Could you check a few things on this model? Use its own coordinates, in mm. A direction names the side the tool comes from. Coordinates: 2 decimals unless noted, no trailing zeros. Write each loop counter-clockwise with the first axis right and the second up, starting at its lowest first coordinate (ties: lowest second). Pieces come first, ordered by that corner, then holes. Notation, with made-up numbers: (-16, 19) - (-11, 19) arc R22 ccw to (-11, 31) - close; hole circle Ø6 at (73, -1). An arc over 180 degrees is marked (long way). Write item = value, one per line. Start each with the question number.
```python
from build123d import *

# Parameters (mm, degrees)
SKETCH1_W           = 40
SKETCH1_H           = 40
BOSS_EXTRUDE1_DEPTH = 40
SKETCH2_W           = 10
SKETCH2_H           = 20
CUT_EXTRUDE1_DEPTH  = 40
CUT_EXTRUDE2_DEPTH  = 40
CUT_EXTRUDE3_DEPTH  = 40
CUT_EXTRUDE4_DEPTH  = 20
CUT_EXTRUDE5_DEPTH  = 10


with BuildPart() as part:
    # Sketch1 → Boss-Extrude1 (new body)
    with BuildSketch(Plane.XY):
        with Locations((20, 20)):
            Rectangle(SKETCH1_W, SKETCH1_H)
    extrude(amount=BOSS_EXTRUDE1_DEPTH)

    # Sketch2 → Cut-Extrude1 (cut)
    with BuildSketch(Plane.XY.offset(40)):
        with Locations((5, 30)):
            Rectangle(SKETCH2_W, SKETCH2_H)
    extrude(amount=-CUT_EXTRUDE1_DEPTH, mode=Mode.SUBTRACT)

    # Sketch3 → Cut-Extrude2 (cut)
    with BuildSketch(Plane.ZY.offset(-10)):
        with BuildLine():
            Line((0, 40), (0, 20))
            ThreePointArc((0, 20), (5.857864376, 34.142135624), (20, 40))
            Line((20, 40), (0, 40))
        make_face()
        with BuildLine():
            Line((40, 40), (20, 40))
            ThreePointArc((20, 40), (34.142135624, 34.142135624), (40, 20))
            Line((40, 20), (40, 40))
        make_face()
    extrude(amount=-CUT_EXTRUDE2_DEPTH, mode=Mode.SUBTRACT)

    # Sketch4 → Cut-Extrude3 (cut)
    with BuildSketch(Plane.ZY):
        with BuildLine():
            ThreePointArc((20, 0), (5.857864376, 5.857864376), (0, 20))
            Line((0, 20), (0, 0))
            Line((0, 0), (20, 0))
        make_face()
        with BuildLine():
            ThreePointArc((40, 20), (34.142135624, 5.857864376), (20, 0))
            Line((20, 0), (40, 0))
            Line((40, 0), (40, 20))
        make_face()
    extrude(amount=-CUT_EXTRUDE3_DEPTH, mode=Mode.SUBTRACT)

    # Sketch5 → Cut-Extrude4 (cut)
    with BuildSketch(Plane.ZY):
        with BuildLine():
            Line((20, 0), (20, 20))
            Line((20, 20), (40, 20))
            ThreePointArc((40, 20), (34.142135624, 5.857864376), (20, 0))
        make_face()
    extrude(amount=-CUT_EXTRUDE4_DEPTH, mode=Mode.SUBTRACT)

    # Sketch6 → Cut-Extrude5 (cut)
    with BuildSketch(Plane(origin=(40, 0, 0), x_dir=(0, 0, -1), z_dir=(1, 0, 0))):
        with BuildLine():
            Line((-20, 40), (-20, 0))
            ThreePointArc((-20, 0), (-40, 20), (-20, 40))
        make_face()
    extrude(amount=-CUT_EXTRUDE5_DEPTH, mode=Mode.SUBTRACT)


solid = part.part
```
1) Suppose I cut it at D-D on z = 4. Please give me the cut outline in (x, y), plus the area to 3 significant figures.
2) Suppose I cut it at A-A on z = 32. Please give me the cut outline in (x, y).
3) If I drill on probe 1 along X at (y, z) = (19, 38.5); probe 2 along Z at (x, y) = (13, 19.5); probe 3 along X at (y, z) = (31, 9.5), over which ranges is the centre line in solid material (lowest first)? Write a range as [from, to].
4) Suppose I cut it at B-B on x = 33.5. Please give me the cut outline in (y, z), plus the area to 3 significant figures.
5) Which directions (+Z, -Z, +X, -X, +Y, -Y) give clear straight access to the entire face, cutting with the end or side of a thin tool? Please do faces 1 (the flat face through (20, 12, 28)), 2 (the flat face through (10, 28, 20)), 3 (the flat face through (0, 12, 12)), 4 (the flat face through (30, 20, 28)), 5 (the flat face through (40, 20, 12)).
6) Suppose I cut it at C-C on y = 13. Please give me the cut outline in (x, z) (3 decimals).
7) For P1, Ø1.5, axis at y = 32.5, z = 23, coming from the +X side; P2, Ø5, axis at x = 14.5, z = 26, coming from the -Y side; P3, Ø6, axis at y = 11, z = 31, coming from the -X side, each with a flat end and sliding along its axis, tell me the tip position at first contact or that it passes through.
Reply:
q1.outline = (0, 8) - (40, 8) - (40, 32) - (10, 32) - (10, 20) - (0, 20) - close
q1.area = 840 mm^2
q2.outline = (10, 20) - (20, 20) - (20, 4) - (30, 4) - (30, 36) - (10, 36) - close
q3.probe_1 = [20, 30]
q3.probe_2 = [0.01, 20]
q3.probe_3 = [10, 40]
q4.outline = (0, 20) arc R20 ccw to (40, 20) - close
q4.area = 628 mm^2
q5.face_1 = +Z, -X, -Y
q5.face_2 = +Z, -Z, -X, +Y
q5.face_3 = +Z, -Z, -X, +Y, -Y
q5.face_4 = +Z, +X, +Y, -Y
q5.face_5 = +Z, -Z, +X, +Y, -Y
q6.outline = (0, 1.265) - (40, 1.265) - (40, 20) - (30, 20) - (30, 38.735) - (20, 38.735) - (20, 20) - (0, 20) - close
q7.P1 = 30
q7.P2 = 20
q7.P3 = 20
